from build123d import *

# Parameters (mm, degrees)
SKETCH1_R           = 3
SKETCH1_R_2         = 2.5
BOSS_EXTRUDE1_DEPTH = 8


with BuildPart() as part:
    # Sketch1 → Boss-Extrude1 (new body)
    with BuildSketch(Plane.XY):
        with BuildLine():
            Line((4, 18), (4, 71))
            ThreePointArc((4, 71), (-0.697580374, 85.722212416), (-4, 70.625695453))
            Line((-4, 70.625695453), (-4, 17.625695453))
            ThreePointArc((-4, 17.625695453), (0.697580374, 2.903483037), (4, 18))
        make_face()
        with Locations((-0.323684855, 77.730954559)):
            Circle(SKETCH1_R, mode=Mode.SUBTRACT)
        with Locations((0.323684855, 10.894740894)):
            Circle(SKETCH1_R_2, mode=Mode.SUBTRACT)
        with BuildLine():
            Line((-2, 69.625695453), (-2, 18.625695453))
            ThreePointArc((-2, 18.625695453), (-1.707106781, 17.918588672), (-1, 17.625695453))
            Line((-1, 17.625695453), (1, 17.625695453))
            ThreePointArc((1, 17.625695453), (1.707106781, 17.918588672), (2, 18.625695453))
            Line((2, 18.625695453), (2, 69.625695453))
            ThreePointArc((2, 69.625695453), (1.707106781, 70.332802234), (1, 70.625695453))
            Line((1, 70.625695453), (-1, 70.625695453))
            ThreePointArc((-1, 70.625695453), (-1.707106781, 70.332802234), (-2, 69.625695453))
        make_face(mode=Mode.SUBTRACT)
    extrude(amount=BOSS_EXTRUDE1_DEPTH)


solid = part.part
Can you work these out from the model? Positions are in its coordinate system, mm. A direction names the side the tool comes from. Coordinates: 2 decimals unless noted, no trailing zeros. Loops run counter-clockwise (first coordinate to the right, second up) from the corner with the lowest first, then second, coordinate; pieces in that order, holes last. Notation, with made-up numbers: (-18, 80.5) - (-6, 80.5) arc R15 ccw to (-6, 103.5) - close; hole circle Ø5 at (-17.75, 77.25). An arc over 180 degrees is marked (long way). Answer as a JSON object with one key per item and string values. Group by question number.
Item 1: If we mould it in two halves opening along X, with no side actions, what happens to faces 4 (the face through (-2, 44, 4)), 5 (the face through (-4, 44, 4)), 6 (the face through (3.6, 44.9, 0))? For each: released by +X, released by -X, zero draft, split by the parting line, or undercut.
Item 2: If I drill on L1, parallel to X at y = 51, z = 1.25; L2, parallel to Y at x = -1.75, z = 7.25; L3, parallel to Y at x = 1.5, z = 7, over which ranges is the centre line in solid material (lowest first)? Write a range as from..to.
Item 3: If we section it at C-C (z = 5.25): List the corners of the cut face in (x, y) for me.
Item 4: For pin 1 (2.5 mm diameter, centred on y = 56, z = 3, fed in from +X); pin 2 (2 mm diameter, centred on y = 40, z = 2, fed in from -X), each with a flat end and sliding along its axis, tell me the tip position at first contact or that it passes through.
Item 5: If we section it at B-B (x = -5.25): List the corners of the cut face in (y, z) for me.
Item 6: On a 3-axis mill with a long thin cutter (end or side, diameter ignored), from which of +Z, -Z, +X, -X, +Y, -Y can I reach the whole of each face in a straight line? I mean faces 1 (the face through (3.6, 44.9, 8)), 2 (the face through (4, 44, 4)), 3 (the face through (0, 17.626, 4)). Say none if no direction works.
Item 7: If we section it at A-A (y = 38): List the corners of the cut face in (x, z) for me.
Returned:
{
 "1": {"face 4": "undercut", "face 5": "released by -X", "face 6": "zero draft"},
 "2": {"L1": "x = -4..-2, 2..4", "L2": "y = 3.17..9.5, 12.29..17.96, 70.29..75.09, 80.37..85.6", "L3": "y = 2.98..8.69, 13.1..17.76, 70.49..75.35, 80.11..85.52"},
 "3": {"outline": "(-4, 17.63) arc R8 ccw (long way) to (4, 18) - (4, 71) arc R8 ccw (long way) to (-4, 70.63) - close; hole circle Ø6 at (-0.32, 77.73); hole circle Ø5 at (0.32, 10.89); hole (-2, 18.63) arc R1 ccw to (-1, 17.63) - (1, 17.63) arc R1 ccw to (2, 18.63) - (2, 69.63) arc R1 ccw to (1, 70.63) - (-1, 70.63) arc R1 ccw to (-2, 69.63) - close"},
 "4": {"pin 1": "stops at x = 4", "pin 2": "stops at x = -4"},
 "5": {"outline": "(5.16, 0) - (16.63, 0) - (16.63, 8) - (5.16, 8) - close; (71.43, 0) - (84.03, 0) - (84.03, 8) - (71.43, 8) - close"},
 "6": {"face 1": "+Z, +X, -X, +Y, -Y", "face 2": "+Z, -Z, +X", "face 3": "+Z, -Z"},
 "7": {"outline": "(-4, 0) - (-2, 0) - (-2, 8) - (-4, 8) - close; (2, 0) - (4, 0) - (4, 8) - (2, 8) - close"}
}
